from build123d import *

# Parameters (mm, degrees)
SKETCH1_W            = 35
SKETCH1_H            = 105
BOSS_EXTRUDE1_DEPTH  = 6
M4_CLEARANCE_HOLE1_D = 4.8
LPATTERN2_COUNT      = 2
LPATTERN2_PITCH      = 10
SKETCH5_W            = 4.8
SKETCH5_H            = 10
SKETCH5_W_2          = 4.730666207
SKETCH5_H_2          = 10.572708501
CUT_EXTRUDE1_DEPTH   = 88.085432636
SKETCH6_W            = 10.8
SKETCH6_H            = 10.8
CUT_EXTRUDE2_DEPTH   = 4
SKETCH7_W            = 6.531210434
SKETCH7_H            = 6.251826861
CUT_EXTRUDE3_DEPTH   = 87.970527062
SKETCH8_W            = 15.98460087
SKETCH8_H            = 8
CUT_EXTRUDE4_DEPTH   = 4
FILLET1_R            = 10
CUT_EXTRUDE5_START   = -6
SKETCH9_W            = 37.049954943
SKETCH9_H            = 41.2
CUT_EXTRUDE5_DEPTH   = 3
FILLET2_R            = 30
FILLET3_R            = 30


with BuildPart() as part:
    # Sketch1 → Boss-Extrude1 (new body)
    with BuildSketch(Plane(origin=(0, 0, 0), x_dir=(1, 0, 0), z_dir=(0, 1, 0))):
        with Locations((0.111940299, -32.574626866)):
            Rectangle(SKETCH1_W, SKETCH1_H)
    extrude(amount=BOSS_EXTRUDE1_DEPTH)

    # M4 Clearance Hole1 (through all)
    with Locations(Plane(origin=(0, 6, 0), x_dir=(1, 0, 0), z_dir=(0, 1, 0))):
        with Locations((-12.388059701, 14.925373134), (12.611940299, 14.925373134), (12.611940299, -10.074626866), (-12.388059701, -10.074626866)):
            m4_clearance_hole1 = Hole(M4_CLEARANCE_HOLE1_D / 2)

    # LPattern2: M4 Clearance Hole1 ×2
    with Locations(*[(0, 0, i * LPATTERN2_PITCH) for i in range(1, LPATTERN2_COUNT)]):
        add(m4_clearance_hole1, mode=Mode.SUBTRACT)

    # Sketch5 → Cut-Extrude1 (cut, through all)
    with BuildSketch(Plane(origin=(0, 6, 0), x_dir=(1, 0, 0), z_dir=(0, 1, 0))):
        with Locations((-12.388059701, 9.925373134)):
            Rectangle(SKETCH5_W, SKETCH5_H)
        with Locations((-12.388059701, -15.074626866)):
            Rectangle(SKETCH5_W, SKETCH5_H)
        with Locations((12.577273403, 9.639018884)):
            Rectangle(SKETCH5_W_2, SKETCH5_H_2)
        with Locations((12.577273403, -15.360981116)):
            Rectangle(SKETCH5_W_2, SKETCH5_H_2)
    extrude(amount=-CUT_EXTRUDE1_DEPTH, mode=Mode.SUBTRACT)

    # Sketch6 → Cut-Extrude2 (cut)
    with BuildSketch(Plane(origin=(0, 6, 0), x_dir=(1, 0, 0), z_dir=(0, 1, 0))):
        with Locations((-0.288059701, -74.674626866)):
            Rectangle(SKETCH6_W, SKETCH6_H)
    extrude(amount=-CUT_EXTRUDE2_DEPTH, mode=Mode.SUBTRACT)

    # Sketch7 → Cut-Extrude3 (cut, through all)
    with BuildSketch(Plane(origin=(0, 2, 0), x_dir=(1, 0, 0), z_dir=(0, 1, 0))):
        with Locations((0, -74.674626866)):
            Rectangle(SKETCH7_W, SKETCH7_H)
    extrude(amount=-CUT_EXTRUDE3_DEPTH, mode=Mode.SUBTRACT)

    # Sketch8 → Cut-Extrude4 (cut)
    with BuildSketch(Plane(origin=(0, 6, 0), x_dir=(1, 0, 0), z_dir=(0, 1, 0))):
        with Locations((-0.195759266, -74.674626866)):
            Rectangle(SKETCH8_W, SKETCH8_H)
    extrude(amount=-CUT_EXTRUDE4_DEPTH, mode=Mode.SUBTRACT)

    # Fillet1
    fillet1_edges = [part.edges().sort_by_distance(p)[0] for p in [
        (17.611940299, 3, 85.074626866),
        (-17.388059701, 3, 85.074626866),
    ]]
    fillet(fillet1_edges, radius=FILLET1_R)

    # Sketch9 → Cut-Extrude5 (cut)
    with BuildSketch(Plane.XZ.offset(CUT_EXTRUDE5_START)):
        with Locations((1.136917771, 64.474626866)):
            Rectangle(SKETCH9_W, SKETCH9_H)
    extrude(amount=CUT_EXTRUDE5_DEPTH, mode=Mode.SUBTRACT)

    # Fillet2
    # the kernel refuses this fillet: 30 mm, written as the material it adds along each edge
    with BuildSketch(Plane(origin=(-17.388059701, 3, 43.874626866), x_dir=(0, 1, 0), z_dir=(1, 0, 0))) as fillet2_piece_1:
        with BuildLine():
            CenterArc((30, 13.076696831), FILLET2_R, 180, 25.841932763)
            Line((0, 13.076696831), (-0.6, 13.076696831))
            Line((-0.6, 13.076696831), (-0.6, 0))
            Line((-0.6, 0), (0, -0.6))
            ThreePointArc((0, -0.6), (1.5, -0.6), (2.46, -0.261533937))
            Line((2.46, -0.261533937), (3, 0))
        make_face()
    extrude(amount=35)

    # Fillet3
    fillet3_edges = [part.edges().sort_by_distance(p)[0] for p in [
        (0.111940299, 6, 43.874626866),
    ]]
    fillet(fillet3_edges, radius=FILLET3_R)


solid = part.part
Build history of the part. All positions in model axes, mm. A direction names the side the tool comes from. Coordinates: 2 decimals unless noted, no trailing zeros. Order: outer loops, then holes, each group sorted by start corner. A loop starts at its lowest first (then second) coordinate and runs counter-clockwise, first axis right, second up. Notation, with made-up numbers: (-35, -24) - (21, -24) arc R19 ccw to (21, -5) - close; hole circle Ø4 at (-21.5, 83.25). An arc over 180 degrees is marked (long way). Write item = value, one per line. Start each with the question number.
1) Saw through at C-C on x = 13. Write the cut outline in (y, z), then the cut area to 3 significant figures.
2) Saw through at B-B on z = -7. Write the cut outline in (x, y), then the cut area to 3 significant figures.
3) Saw through at A-A on x = 2. Write the cut outline in (y, z).
4) Wall check: line 1 along X through (y, z) = (4.1, -7); line 2 along X through (y, z) = (3.6, -3.5); line 3 along Z through (x, y) = (5, 2.5). Give the ranges that are in metal, low to high. Write a range as from..to.
5) Two-plate mould, pull along Z, no slides. Class faces 4 (the face through (14.605, 1.521, 82.223)), 5 (the face through (-12.441, 2.958, -17.325)), 6 (the face through (0, 6, 9)): pulls with the +Z half, pulls with the -Z half, needs draft (parallel to the pull), parting line crosses it, or undercut.
6) Flat gauge pins, fed straight in: pin 1 Ø0.8 at (y, z) = (2.5, 79) entering from -X; pin 2 Ø8.5 at (x, z) = (1, 64) entering from +Y. Where does each tip first touch, or does it go through?
7) 3-axis set-ups, long thin cutter, end or side, ignore diameter. For faces 1 (the face through (0, 0, 32)), 2 (the face through (10.212, 3, -10)), 3 (the face through (0, 3, 68)): which of +Z, -Z, +X, -X, +Y, -Y reach the whole face in a straight line?
8) Saw through at D-D on z = 65. Write the cut outline in (x, y), then the cut area to 3 significant figures.
From the geometry:
q1.outline = (0, -19.93) - (6, -19.93) - (6, -17.29) - (0, -17.29) - close; (0, -2.56) - (6, -2.56) - (6, 7.71) - (0, 7.71) - close; (0, 22.44) - (6, 22.44) - (6, 38.22) arc R30 ccw to (4.5, 47.58) arc R30 cw to (3, 56.95) - (3, 83.5) - (0, 83.5) - close
q1.area = 336 mm^2
q2.outline = (-17.39, 0) - (-14.79, 0) - (-14.79, 6) - (-17.39, 6) - close; (-9.99, 0) - (10.21, 0) - (10.21, 6) - (-9.99, 6) - close; (14.94, 0) - (17.61, 0) - (17.61, 6) - (14.94, 6) - close
q2.area = 153 mm^2
q3.outline = (0, -19.93) - (6, -19.93) - (6, 38.22) arc R30 ccw to (4.5, 47.58) arc R30 cw to (3, 56.95) - (3, 69.27) - (2, 69.27) - (2, 71.55) - (0, 71.55) - close; (0, 77.8) - (2, 77.8) - (2, 80.07) - (3, 80.07) - (3, 85.07) - (0, 85.07) - close
q4.line_1 = -17.39..-14.79, -9.99..10.21, 14.94..17.61
q4.line_2 = -17.39..-14.32, -10.46..10.68, 14.54..17.61
q4.line_3 = -19.93..69.27, 80.07..85.07
q5.face_4 = pulls with the +Z half
q5.face_5 = undercut
q5.face_6 = needs draft
q6.pin_1 = -16.75
q6.pin_2 = 3
q7.face_1 = +Z, -Z, +X, -X, -Y
q7.face_2 = +Y, -Y
q7.face_3 = +Z, +X, -X, +Y
q8.outline = (-17.39, 0) - (17.61, 0) - (17.61, 3) - (-17.39, 3) - close
q8.area = 105 mm^2
